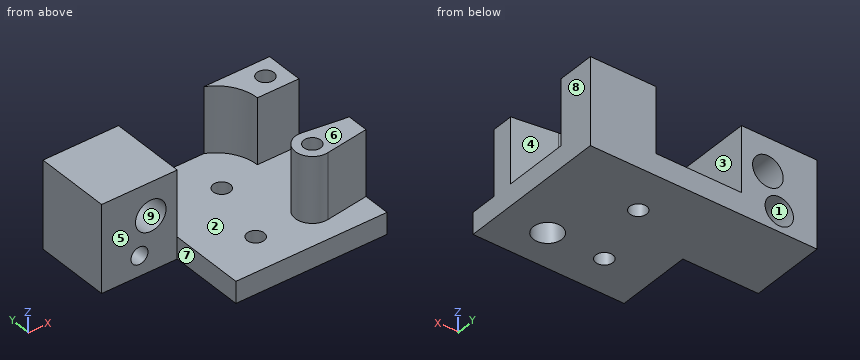
```python
from build123d import *

# Parameters (mm, degrees)
SKETCH_R        = 2.25
PAD_DEPTH       = 23
POCKET_DEPTH    = 17.3
SKETCH002_R     = 4.05
SKETCH002_R_2   = 2.25
POCKET001_DEPTH = 20.001
SKETCH003_R     = 2.25
POCKET002_DEPTH = 10
SKETCH004_R     = 3.75
POCKET003_DEPTH = 10
SKETCH005_R     = 3.75
POCKET004_DEPTH = 9.2


with BuildPart() as part:
    # Sketch → Pad (new body)
    with BuildSketch(Plane.XY):
        Polygon((0, -20), (40, -20), (40, 20), (-20, 20), (-20, 0), (0, 0), align=None)
        with Locations((18, 8)):
            Circle(SKETCH_R, mode=Mode.SUBTRACT)
        with Locations((13, -10)):
            Circle(SKETCH_R, mode=Mode.SUBTRACT)
        with Locations((28, -10)):
            Circle(SKETCH_R, mode=Mode.SUBTRACT)
    extrude(amount=PAD_DEPTH)

    # Sketch001 → Pocket (cut)
    with BuildSketch(Plane.XY.offset(23)):
        with BuildLine():
            Line((46, 10), (29, 10))
            ThreePointArc((29, 10), (25.778159, 17.77819), (17.999956, 21))
            Line((17.999956, 21), (0, 21))
            Line((0, 21), (0, -23))
            Line((0, -23), (46, -23))
            Line((46, -23), (46, -12))
            Line((28.629923, -14.455693), (46, -12))
            ThreePointArc((28.629923, -5.544307), (23.5, -10), (28.629923, -14.455693))
            Line((28.629923, -5.544307), (46, -8))
            Line((46, -8), (46, 10))
        make_face()
    extrude(amount=-POCKET_DEPTH, mode=Mode.SUBTRACT)

    # Sketch002 → Pocket001 (cut, through all)
    with BuildSketch(Plane.XZ):
        with Locations((-7, 14.3)):
            Circle(SKETCH002_R)
        with Locations((-10, 5.3)):
            Circle(SKETCH002_R_2)
    extrude(amount=-POCKET001_DEPTH, mode=Mode.SUBTRACT)

    # Sketch003 → Pocket002 (cut)
    with BuildSketch(Plane.XY.offset(23)):
        with Locations((35, 15)):
            Circle(SKETCH003_R)
    extrude(amount=-POCKET002_DEPTH, mode=Mode.SUBTRACT)

    # Sketch004 → Pocket003 (cut)
    with BuildSketch(Plane(origin=(0, 20, 0), x_dir=(-1, 0, 0), z_dir=(0, 1, 0))):
        with Locations((10, 5.3)):
            Circle(SKETCH004_R)
    extrude(amount=-POCKET003_DEPTH, mode=Mode.SUBTRACT)

    # Sketch005 → Pocket004 (cut)
    with BuildSketch(Plane(origin=(0, 0, 0), x_dir=(1, 0, 0), z_dir=(0, 0, -1))):
        with Locations((28, 10)):
            Circle(SKETCH005_R)
    extrude(amount=-POCKET004_DEPTH, mode=Mode.SUBTRACT)


solid = part.part
```
Input: part model. Units: mm. Frame: model coordinates. Face numbers are marked on the shaded views. A direction names the side the tool comes from. Coordinates: 2 decimals unless noted, no trailing zeros. Order: outer loops, then holes, each group sorted by start corner. A loop starts at its lowest first (then second) coordinate and runs counter-clockwise, first axis right, second up. Notation, with made-up numbers: (37, -18) - (62, -18) arc R16 ccw to (62, 12) - close; hole circle Ø9 at (55.25, 58.5). An arc over 180 degrees is marked (long way). Put each result on its own line as item: value.
1. Cut plane A-A on z = 20. Return the cut outline in (x, y).
Report:
outline: (-20, 0) - (0, 0) - (0, 20) - (-20, 20) - close; (22.58, 20) arc R11 cw to (29, 10) - (40, 10) - (40, 20) - close; (28.63, -14.46) - (40, -12.85) - (40, -7.15) - (28.63, -5.54) arc R4.5 ccw (long way) to start; hole circle Ø4.5 at (28, -10); hole circle Ø4.5 at (35, 15)
2. Line query: line 1 along Z through (x, y) = (-7, 16.25); line 2 along X through (y, z) = (-10, 17.5); line 3 along Y through (x, z) = (27, 13). Output: solid intervals per line, ascending.
Report:
line 1: z = 0 to 3.05, 7.55 to 10.25, 18.35 to 23
line 2: x = 23.5 to 25.75, 30.25 to 40
line 3: y = -14.39 to -12.02, -7.98 to -5.61, 16.32 to 20
3. Cut plane D-D on z = 14.3. Return the cut outline in (x, y), then the cut area to 3 significant figures.
Report:
outline: (-20, 0) - (-11.05, 0) - (-11.05, 20) - (-20, 20) - close; (-2.95, 0) - (0, 0) - (0, 20) - (-2.95, 20) - close; (22.58, 20) arc R11 cw to (29, 10) - (40, 10) - (40, 20) - close; (28.63, -14.46) - (40, -12.85) - (40, -7.15) - (28.63, -5.54) arc R4.5 ccw (long way) to start; hole circle Ø4.5 at (28, -10); hole circle Ø4.5 at (35, 15)
area: 455 mm2
4. Contact query for flat-ended pins moving along their axis: pin 1 Ø2.5 at (x, y) = (18, 8) entering from -Z; pin 2 Ø13 at (x, z) = (-7, 14.3) entering from -Y; pin 3 Ø4 at (x, y) = (8, 10.5) entering from -Z; pin 4 Ø8 at (x, y) = (11, -15) entering from +Z. Output: stop coordinate, or through.
Report:
pin 1: passes through
pin 2: stops at y = 0
pin 3: stops at z = 0
pin 4: stops at z = 5.7
5. Cut plane B-B on x = 18. Return the cut outline in (y, z).
Report:
outline: (-20, 0) - (5.75, 0) - (5.75, 5.7) - (-20, 5.7) - close; (10.25, 0) - (20, 0) - (20, 5.7) - (10.25, 5.7) - close
6. Reachability of the marked faces 1, 2, 3, 4 and 5 from +Z, -Z, +X, -X, +Y, -Y: full face, straight path, thin tool, end or side. Return the list, or none.
Report:
face 1: +Y
face 2: +Z
face 3: +Z, +Y, -Y
face 4: +Z, +X
face 5: +Z, -Z, -X, -Y
7. Cut plane C-C on y = -10. Return the cut outline in (x, z), then the cut area to 3 significant figures.
Report:
outline: (0, 0) - (10.75, 0) - (10.75, 5.7) - (0, 5.7) - close; (15.25, 0) - (24.25, 0) - (24.25, 9.2) - (25.75, 9.2) - (25.75, 23) - (23.5, 23) - (23.5, 5.7) - (15.25, 5.7) - close; (30.25, 9.2) - (31.75, 9.2) - (31.75, 0) - (40, 0) - (40, 23) - (30.25, 23) - close
area: 357 mm2
8. Draft query along X for the marked faces 6, 7, 8 and 9. Return one class per face: pulls with the +X half, pulls with the -X half, needs draft (parallel to the pull), parting line crosses it, or undercut.
Report:
face 6: needs draft
face 7: pulls with the -X half
face 8: pulls with the +X half
face 9: undercut
